Here's how the part is built. I have some questions about the finished solid (model axes, mm). Round coordinates to 2 decimals unless told otherwise and drop trailing zeros. Loops run counter-clockwise (first coordinate to the right, second up) from the corner with the lowest first, then second, coordinate; pieces in that order, holes last. Notation, with made-up numbers: M 45.25,-13 L 89.25,-13 A14 cw 89.25,12 Z; hole C 2,45.5 d10. An arc over 180 degrees is marked long. Answer as CSV lines item,"result".
Autodesk Inventor part; units mm, degrees
ref_plane "YZ Plane" through (0, 0, 0) normal (1, 0, 0) x (0, 1, 0)
ref_plane "XZ Plane" through (0, 0, 0) normal (0, 1, 0) x (-1, 0, 0)
ref_plane "XY Plane" through (0, 0, 0) normal (0, 0, 1) x (1, 0, 0)
sketch "Sketch1" plane through (0, 0, 0) normal (0, 1, 0) x (-1, 0, 0)
  line L0 (-259.8076, 150) -> (-259.8076, 90)
  line L1 (-259.8076, 90) -> (-51.9615, -30)
  line L2 (-51.9615, -30) -> (0, 0)
  line L3 (0, 0) -> (0, 240)
  line L4 (0, 240) -> (-51.9615, 270)
  line L5 (-51.9615, 270) -> (-259.8076, 150)
  dimension "d0" = 120
  dimension "d1" = 120
  dimension "d2" = 120
  dimension "d4" = 120
  dimension "d5" = 120
  dimension "d6" = 60
  dimension "d7" = 120
  dimension "d71" = 259.8076
  dimension "d72" = 300
extrude "Extrusion1" add sketch "Sketch1" along normal blind 5
sketch "Sketch2" plane through (0, 5, 0) normal (0, 1, 0) x (1, 0, 0)
  line L0 (254.8076, -108) -> (254.8076, -132)
  line L1 (259.8076, -150) -> (259.8076, -90)
  line L2 (259.8076, -90) -> (51.9615, 30)
  line L3 (51.9615, -270) -> (259.8076, -150)
  line L4 (209.8076, -108) -> (209.8076, -132)
  line L5 (209.8076, -108) -> (209.8076, -100)
  line L6 (209.8076, -144.7569) -> (209.8076, -140)
  point P0 (0, 0)
  dimension "d10" = 24
  dimension "d11" = 5
  dimension "d12" = 18
  dimension "d31" = 18.0885
  dimension "d32" = 18.0885
  dimension "d33" = 18
  dimension "d44" = 45
  dimension "d45" = 0
  dimension "d47" = 40.5885
  dimension "d51" = 8
  dimension "d52" = 8
hole "Hole1" at (209.8076, 5, 100) at (209.8076, 5, 140) at (254.8076, 5, 108) at (254.8076, 5, 132) direction (0, -1, 0) diameter 2.8 end through all
sketch "Sketch3" plane through (0, 5, 0) normal (0, 1, 0) x (1, 0, 0)
  line L0 (18.088, 4.6696) -> (38.8735, 16.6701)
  line L1 (51.9615, 30) -> (0, 0)
  line L2 (0, 0) -> (0, -240)
  line L3 (259.8076, -90) -> (51.9615, 30)
  line L4 (51.413, -28.0517) -> (72.1985, -16.0512)
  line L5 (72.1985, -16.0512) -> (68.3015, -18.3011)
  line L6 (51.413, -28.0517) -> (33.66, -38.3014)
  dimension "d20" = 5
  dimension "d22" = 18.088
  dimension "d23" = 18.088
  dimension "d46" = 45
  dimension "d53" = 33.66
  dimension "d73" = 33.66
hole "Hole2" at (68.3015, 5, 18.3011) at (33.66, 5, 38.3014) at (18.088, 5, -4.6696) at (38.8735, 5, -16.6701) direction (0, -1, 0) diameter 2.8 end through all
sketch "Sketch4" plane through (0, 5, 0) normal (0, 1, 0) x (1, 0, 0)
  line L0 (18.088, -244.6696) -> (38.8735, -256.6701)
  line L1 (0, -240) -> (51.9615, -270)
  line L2 (51.9615, -270) -> (259.8076, -150)
  line L3 (0, 0) -> (0, -240)
  line L4 (47.516, -209.6983) -> (68.3015, -221.6989)
  line L5 (68.3015, -221.6989) -> (68.3015, -221.6989)
  line L6 (25.866, -197.1987) -> (33.66, -201.6986)
  dimension "d34" = 5
  dimension "d35" = 18.088
  dimension "d36" = 18.088
  dimension "d49" = 45
  dimension "d74" = 33.66
  dimension "d75" = 33.66
  dimension "d76" = 33.66
hole "Hole3" at (68.3015, 5, 221.6989) at (33.66, 5, 201.6986) at (18.088, 5, 244.6696) at (38.8735, 5, 256.6701) direction (0, -1, 0) diameter 2.8 end through all
sketch "Sketch5" plane through (0, 0, 0) normal (0, -1, 0) x (1, 0, 0)
  circle A0 centre (18.088, 244.6696) radius 1.4
  circle A1 centre (68.3015, 221.6989) radius 1.4
  circle A2 centre (33.66, 201.6986) radius 1.4
  circle A3 centre (38.8735, 256.6701) radius 1.4
  circle A4 centre (18.088, -4.6696) radius 1.4
  circle A5 centre (68.3015, 18.3011) radius 1.4
  circle A6 centre (33.66, 38.3014) radius 1.4
  circle A7 centre (38.8735, -16.6701) radius 1.4
  circle A8 centre (254.8076, 108) radius 1.4
  circle A9 centre (209.8076, 100) radius 1.4
  circle A10 centre (209.8076, 140) radius 1.4
  circle A11 centre (254.8076, 132) radius 1.4
  line L0 (259.8076, 90) -> (51.9615, -30)
  line L1 (259.8076, 150) -> (259.8076, 90)
  line L2 (51.9615, 270) -> (259.8076, 150)
  line L3 (0, 240) -> (51.9615, 270)
  line L4 (0, 0) -> (0, 240)
  line L5 (51.9615, -30) -> (0, 0)
  circle A12 centre (254.8076, 108) radius 1.4
  circle A13 centre (254.8076, 108) radius 3
  circle A14 centre (254.8076, 132) radius 1.4
  circle A15 centre (254.8076, 132) radius 3
  circle A16 centre (209.8076, 100) radius 3
  circle A17 centre (209.8076, 140) radius 3
  circle A18 centre (68.3015, 221.6989) radius 1.4
  circle A19 centre (68.3015, 221.6989) radius 3
  circle A20 centre (38.8735, 256.6701) radius 1.4
  circle A21 centre (38.8735, 256.6701) radius 3
  circle A22 centre (18.088, 244.6696) radius 1.4
  circle A23 centre (18.088, 244.6696) radius 3
  circle A24 centre (33.66, 201.6986) radius 3
  circle A25 centre (33.66, 38.3014) radius 1.4
  circle A26 centre (33.66, 38.3014) radius 3
  circle A27 centre (68.3015, 18.3011) radius 1.4
  circle A28 centre (68.3015, 18.3011) radius 3
  circle A29 centre (38.8735, -16.6701) radius 1.4
  circle A30 centre (38.8735, -16.6701) radius 3
  circle A31 centre (18.088, -4.6696) radius 1.4
  circle A32 centre (18.088, -4.6696) radius 3
  dimension "d57" = 6
  dimension "d58" = 6
  dimension "d59" = 6
  dimension "d60" = 6
  dimension "d61" = 6
  dimension "d62" = 6
  dimension "d63" = 6
  dimension "d64" = 6
  dimension "d65" = 6
  dimension "d66" = 6
  dimension "d67" = 6
  dimension "d68" = 6
extrude "Extrusion2" cut sketch "Sketch5" against normal blind 2.3 contours A13 | A15 | A16 | A17 | A19 | A21 | A23 | A24 | A26 | A28 | A30 | A32
properties part number "lap" material "Wood (Birch)"
1. I want a section at C-C, the plane x = 133.5. Please give me the cut outline in (y, z), and give its area (3 significant figures).
Evaluation:
outline,"M 0,17.08 L 5,17.08 L 5,222.92 L 0,222.92 Z"
area,"1,030 mm²"
2. For P1, Ø1, axis at x = 54.5, y = 3, coming from the -Z side; P2, Ø3, axis at x = 34.5, z = 39, coming from the -Y side; P3, Ø1.7, axis at x = 18.09, z = -4.67, coming from the +Y side, each with a flat end and sliding along its axis, tell me the tip position at first contact or that it passes through.
Evaluation:
P1,"stops at z = -28.82"
P2,"stops at y = 2.3"
P3,"passes through"
3. I want a section at B-B, the plane x = 183. Please give me the cut outline in (y, z), and give its area (3 significant figures).
Evaluation:
outline,"M 0,45.66 L 5,45.66 L 5,194.34 L 0,194.34 Z"
area,"743 mm²"
4. We'd pull the mould along Z, two halves only. Please class faces 1 (the flat face through (103, 5, 122)), 2 (the flat face through (154.43, 2.46, 210.84)), 3 (the flat face through (157.34, 2.46, 30.84)), 4 (the cylindrical face through (17.44, 1.13, 241.74)): pulls with the +Z half, pulls with the -Z half, needs draft (parallel to the pull), parting line crosses it, or undercut.
Evaluation:
face 1,"needs draft"
face 2,"pulls with the +Z half"
face 3,"pulls with the -Z half"
face 4,"undercut"
5. If I drill on line 1 (X direction, y = 4.35, z = 108); line 2 (Z direction, x = 212, y = 1); line 3 (Z direction, x = 72.5, y = 4.1), over which ranges is the centre line in solid material (lowest first)? Write a range as [from, to].
Evaluation:
line 1,"x = [0, 253.41], [256.21, 259.81]"
line 2,"z = [62.4, 97.95], [102.05, 137.95], [142.05, 177.6]"
line 3,"z = [-18.14, 258.14]"
6. I want a section at A-A, the plane y = 1.5. Count the separate pieces of the cut face and the enclosed holes in it, and give its area (3 significant figures).
Evaluation:
separate pieces,"1"
enclosed holes,"12"
area,"51,100 mm²"
